The model under review builds one solid part; all positions refer to its coordinate system, in mm. Give positions to 0.01 mm unless a question says otherwise; leave off trailing zeros. Loops run counter-clockwise (first coordinate to the right, second up) from the corner with the lowest first, then second, coordinate; pieces in that order, holes last. Notation, with made-up numbers: M 20,-17.5 L 51,-17.5 A30 cw 51,7.5 Z; hole C -28,40.5 d4. An arc over 180 degrees is marked long. Put each result on its own line as item: value. Start each with the question number.
```python
from build123d import *

# Parameters (mm, degrees)
F0_W           = 372
F0_H           = 280
F1_DEPTH       = 6
F2_R           = 25
F3_DEPTH       = 6
F5_D           = 3.4
F9_D           = 2.5
F9_DEPTH       = 16.5
F9_TIP         = 0.7510757738
F9_ON_F8_D     = 2.5
F9_ON_F8_DEPTH = 16.5
F9_ON_F8_TIP   = 0.7510757738
F9_ON_F7_D     = 2.5
F9_ON_F7_DEPTH = 16.5
F9_ON_F7_TIP   = 0.7510757738
F10_D          = 2.5
F10_DEPTH      = 16.5
F10_TIP        = 0.7510757738


# Not quite as in the source:
# - a feature names something its author has since deleted; it is built from what else it names


with BuildPart() as f1:
    # F0 (on Top) → F1 (new body)
    with BuildSketch(Plane.XY):
        Rectangle(F0_W, F0_H)
    extrude(amount=F1_DEPTH)


with BuildPart() as f3:
    # F2 (on face) → F3 (new body)
    with BuildSketch(Plane.XY.offset(6)):
        with Locations((-116, 60)):
            Circle(F2_R)
    extrude(amount=-F3_DEPTH)


with BuildPart() as f1_1:
    add(f1.part)

    # F4: cut F3
    add(f3.part, mode=Mode.SUBTRACT)

    # F5 (through all)
    with Locations(Plane.XY.offset(6)):
        with Locations((-116, 94), (-145.4448637287, 43), (-86.5551362713, 43)):
            Hole(F5_D / 2)

    # F9
    with Locations(Plane.YZ.offset(186)):
        with Locations((-100, 3), (0, 3), (100, 3)):
            Hole(F9_D / 2, depth=F9_DEPTH)
            with Locations((0, 0, -(F9_DEPTH + F9_TIP / 2))):  # 118° drill point
                Cone(0, F9_D / 2, F9_TIP, mode=Mode.SUBTRACT)

    # F9 on F8
    with Locations(Plane(origin=(0, 140, 0), x_dir=(-1, 0, 0), z_dir=(0, 1, 0))):
        with Locations((-150, 3), (-50, 3), (50, 3)):
            Hole(F9_ON_F8_D / 2, depth=F9_ON_F8_DEPTH)
            with Locations((0, 0, -(F9_ON_F8_DEPTH + F9_ON_F8_TIP / 2))):  # 118° drill point
                Cone(0, F9_ON_F8_D / 2, F9_ON_F8_TIP, mode=Mode.SUBTRACT)

    # F9 on F7
    with Locations(Plane(origin=(-186, 0, 0), x_dir=(0, -1, 0), z_dir=(-1, 0, 0))):
        with Locations((-100, 3), (0, 3), (100, 3)):
            Hole(F9_ON_F7_D / 2, depth=F9_ON_F7_DEPTH)
            with Locations((0, 0, -(F9_ON_F7_DEPTH + F9_ON_F7_TIP / 2))):  # 118° drill point
                Cone(0, F9_ON_F7_D / 2, F9_ON_F7_TIP, mode=Mode.SUBTRACT)

    # F10
    with Locations(Plane(origin=(0, 140, 0), x_dir=(-1, 0, 0), z_dir=(0, 1, 0))):
        with Locations((150, 3)):
            Hole(F10_D / 2, depth=F10_DEPTH)
            with Locations((0, 0, -(F10_DEPTH + F10_TIP / 2))):  # 118° drill point
                Cone(0, F10_D / 2, F10_TIP, mode=Mode.SUBTRACT)


solid = f1_1.part
```
Item 1: Consider section A-A, the plane y = 60. Write out the cut boundary in (x, z), plus the area to 3 significant figures.
Item 2: Clearance check with flat-ended pins moving along their axes: pin 1 Ø2 at (y, z) = (0, 3) entering from -X; pin 2 Ø2 at (y, z) = (100, 3) entering from +X; pin 3 Ø1.5 at (x, z) = (150, 3) entering from +Y; pin 4 Ø3 at (x, y) = (-116, 94) entering from -Z. State where each tip first meets the part, or that it passes through.
Item 3: To check wall thickness, follow L1, parallel to Y at x = 179.75, z = 3; L2, parallel to Y at x = -116, z = 2.7; L3, parallel to X at y = 129, z = 3. State the ranges of each line that lie inside material, in increasing order. Write a range as [from, to].
Item 4: Draft analysis for pull direction Y (two halves, no side actions). For faces 1 (the flat face through (-3, 2, 0)), 2 (the cylindrical face through (-140.976, 61.099, 3.042)), state which applies: +Y half, -Y half, draft (parallel to the pull), parting line (faces both ways), or undercut.
Report:
1. outline: M -186,0 L -141,0 L -141,6 L -186,6 Z; M -91,0 L 186,0 L 186,6 L -91,6 Z
1. area: 1,930 mm²
2. pin 1: x = -169.35
2. pin 2: x = 169.35
2. pin 3: y = 123.2
2. pin 4: through
3. L1: [-140, -101.25], [-98.75, -1.25], [1.25, 98.75], [101.25, 140]
3. L2: [-140, 35], [85, 92.3], [95.7, 140]
3. L3: [-186, -151.25], [-148.75, -51.25], [-48.75, 48.75], [51.25, 148.75], [151.25, 186]
4. face 1: draft
4. face 2: undercut
